from build123d import *

# Parameters (mm, degrees)
SKETCH1_W           = 20
SKETCH1_H           = 20
SKETCH1_W_2         = 16
SKETCH1_H_2         = 16
BOSS_EXTRUDE1_DEPTH = 460.04
SKETCH2_R           = 4
CUT_EXTRUDE1_DEPTH  = 461.583110415
SKETCH5_R           = 4
CUT_EXTRUDE2_DEPTH  = 461.583110415
LPATTERN1_COUNT     = 6
LPATTERN1_PITCH     = 24.6
SKETCH6_R           = 4
CUT_EXTRUDE3_DEPTH  = 461.583110415


with BuildPart() as part:
    # Sketch1 → Boss-Extrude1 (new body)
    with BuildSketch(Plane.XY):
        Rectangle(SKETCH1_W, SKETCH1_H)
        Rectangle(SKETCH1_W_2, SKETCH1_H_2, mode=Mode.SUBTRACT)
    extrude(amount=BOSS_EXTRUDE1_DEPTH)

    # Sketch2 → Cut-Extrude1 (cut, through all)
    with BuildSketch(Plane(origin=(0, 10, 0), x_dir=(1, 0, 0), z_dir=(0, 1, 0))):
        with Locations(Location((0, -15, 0), (0, 0, 270))):
            Circle(SKETCH2_R)
    cut_extrude1 = extrude(amount=-CUT_EXTRUDE1_DEPTH, mode=Mode.SUBTRACT)

    # Mirror1: Cut-Extrude1 across plane
    add(cut_extrude1.mirror(Plane.XY.offset(230.02)), mode=Mode.SUBTRACT)

    # Sketch5 → Cut-Extrude2 (cut, through all)
    with BuildSketch(Plane(origin=(10, 0, 0), x_dir=(0, 0, -1), z_dir=(1, 0, 0))):
        with Locations(Location((-291.33, 0, 0), (0, 0, 90))):
            Circle(SKETCH5_R)
    cut_extrude2 = extrude(amount=-CUT_EXTRUDE2_DEPTH, mode=Mode.SUBTRACT)

    # LPattern1: Cut-Extrude2 ×6
    with Locations(*[(0, 0, -i * LPATTERN1_PITCH) for i in range(1, LPATTERN1_COUNT)]):
        add(cut_extrude2, mode=Mode.SUBTRACT)

    # Sketch6 → Cut-Extrude3 (cut, through all)
    with BuildSketch(Plane(origin=(0, 10, 0), x_dir=(1, 0, 0), z_dir=(0, 1, 0))):
        with Locations(Location((0, -303.82, 0), (0, 0, 270))):
            Circle(SKETCH6_R)
        with Locations(Location((0, -279.22, 0), (0, 0, 270))):
            Circle(SKETCH6_R)
    cut_extrude3 = extrude(amount=-CUT_EXTRUDE3_DEPTH, mode=Mode.SUBTRACT)

    # Mirror2: Cut-Extrude3 across plane
    add(cut_extrude3.mirror(Plane.XY.offset(230.02)), mode=Mode.SUBTRACT)


solid = part.part
For this review, take the finished solid that the model builds, in its own axes (mm). A direction names the side the tool comes from. Coordinates: 2 decimals unless noted, no trailing zeros. Order: outer loops, then holes, each group sorted by start corner. A loop starts at its lowest first (then second) coordinate and runs counter-clockwise, first axis right, second up. Notation, with made-up numbers: (40.5, 23.25) -> (70.5, 23.25) arc R23 cw to (70.5, 52.25) -> close; hole circle Ø11 at (29, 5.25). An arc over 180 degrees is marked (long way). Return JSON: item names as keys, results as strings.
1. Machinability: for faces 1 (the flat face through (0, -8, 227)), 2 (the cylindrical face through (-1.532, 9.014, 282.915)), which of the approach directions +Z, -Z, +X, -X, +Y, -Y give a long, thin tool a straight path to every point of the face, cutting with its end or side? Answer none if there is none.
Answer block:
{"face 1": "+Z, -Z", "face 2": "+Y, -Y"}
2. For line 1 (Y direction, x = 4.25, z = 397.5); line 2 (Y direction, x = -9.6, z = 266.73), list the stretches that pass through material, from the lowest coordinate up. Write a range as from..to.
Answer block:
{"line 1": "-10..-8, 8..10", "line 2": "-10..-4, 4..10"}
3. We need section B-B on y = 0. State how many separate pieces and enclosed holes the cut face has, and give its area (3 significant figures).
Answer block:
{"separate pieces": "14", "enclosed holes": "0", "area": "1,650 mm²"}
4. For pin 1 Ø5 at (x, z) = (0, 279.22) entering from -Y, flat-tipped, find the tip position at first contact; note if it passes through.
Answer block:
{"pin 1": "through"}
5. The part is to be moulded in two halves that separate along Z. For faces 3 (the flat face through (8, 0, 227)), 4 (the flat face through (-9, 0, 0)), 5 (the flat face through (-9, 0, 460.04)), 6 (the cylindrical face through (-9, -0.5, 295.3)), say which applies: +Z half, -Z half, draft (parallel to the pull), parting line (faces both ways), or undercut.
Answer block:
{"face 3": "draft", "face 4": "-Z half", "face 5": "+Z half", "face 6": "undercut"}
6. We need section A-A on z = 156.22. Write out the cut boundary in (x, y).
Answer block:
{"outline": "(-10, -10) -> (-4, -10) -> (-4, -8) -> (-8, -8) -> (-8, 8) -> (-4, 8) -> (-4, 10) -> (-10, 10) -> close; (4, -10) -> (10, -10) -> (10, 10) -> (4, 10) -> (4, 8) -> (8, 8) -> (8, -8) -> (4, -8) -> close"}
